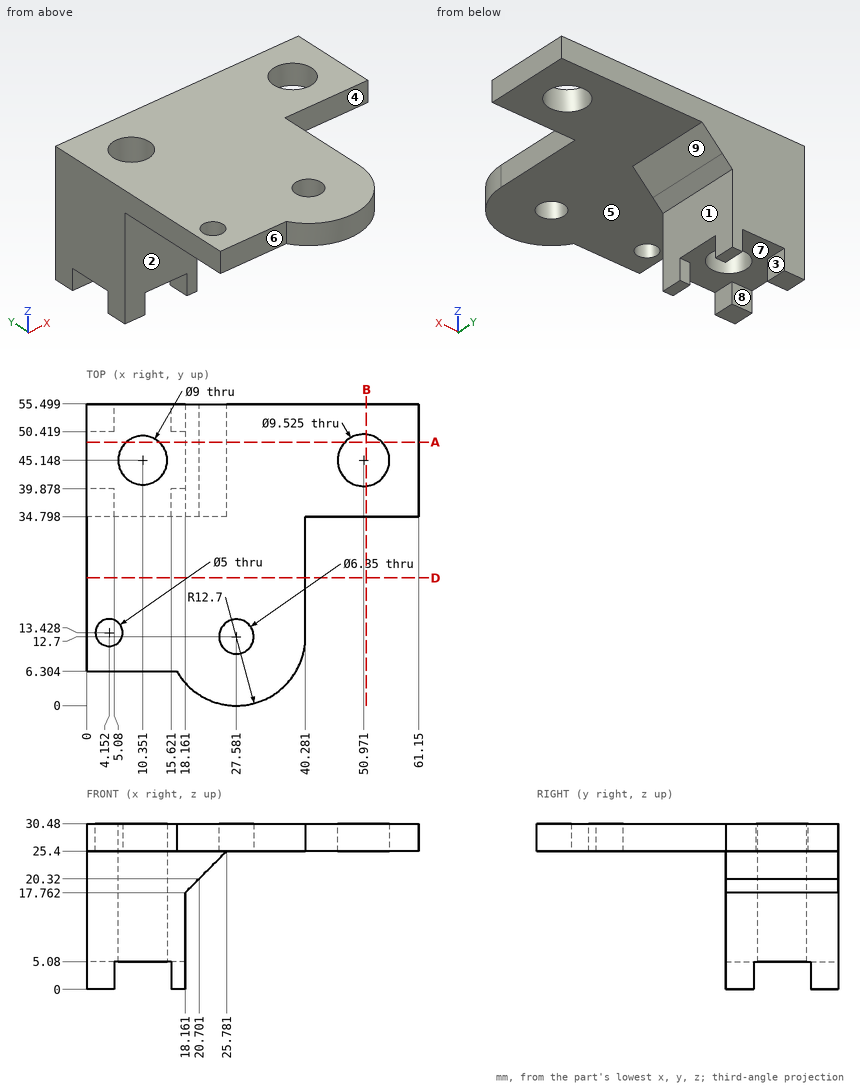
The drawing under review shows one solid part. Ordinate dimensions are in mm from its lowest x, y, z. A direction names the side the tool comes from. Round coordinates to 2 decimals unless told otherwise and drop trailing zeros. Write each loop counter-clockwise with the first axis right and the second up, starting at its lowest first coordinate (ties: lowest second). Pieces come first, ordered by that corner, then holes. Notation, with made-up numbers: M 31,64.25 L 35,64.25 A11 ccw 35,80.25 Z; hole C -8,-23.75 d6. An arc over 180 degrees is marked long. One line per item, written item: value. Start each with the question number.
(1) Insertion check: pin 1 (4 mm diameter, centred on y = 52.5, z = 1.5, fed in from +X); pin 2 (4 mm diameter, centred on x = 2, z = 3.5, fed in from -Y); pin 3 (14.5 mm diameter, centred on x = 10.35, y = 45.15, fed in from -Z); pin 4 (4 mm diameter, centred on x = 4.15, y = 13.43, fed in from +Z). Each pin has a flat end and moves straight along its axis. Give the tip position at first contact, or say it passes through.
(2) Machinability: for the marked faces 1, 2, 3, 4 and 5, which of the approach directions +Z, -Z, +X, -X, +Y, -Y give a long, thin tool a straight path to every point of the face, cutting with its end or side? Answer none if there is none.
(3) Wall thickness on line 1 (Y direction, x = 10, z = 23.5) (1 decimal); line 2 (Z direction, x = 30, y = 24); line 3 (Y direction, x = 30, z = 26) (1 decimal): over which ranges is each line inside the solid? List them lowest first.
(4) We need section D-D (y = 23.5). Give the boundary of the cut face in (x, z), and give its area (3 significant figures).
(5) We need section A-A (y = 48.5). Count the separate pieces of the cut face and the enclosed holes in it, and give its area (3 significant figures).
(6) We need section B-B (x = 51.5). Give the boundary of the cut face in (y, z) (1 decimal).
(7) The part is to be moulded in two halves that separate along Y. For the marked faces 6, 7, 8 and 9, say which applies: released by +Y, released by -Y, zero draft, split by the parting line, or undercut.
Result:
1. pin 1: x = 18.16
1. pin 2: y = 34.8
1. pin 3: z = 5.08
1. pin 4: through
2. face 1: -Z, +X, +Y, -Y
2. face 2: -Z, +X, -X, -Y
2. face 3: -Z, +Y, -Y
2. face 4: +Z, -Z, +X, -Y
2. face 5: -Z, +X, -Y
3. line 1: 34.8 to 40.7, 49.6 to 55.5
3. line 2: 25.4 to 30.48
3. line 3: 0.2 to 10.6, 14.8 to 55.5
4. outline: M 0,25.4 L 40.28,25.4 L 40.28,30.48 L 0,30.48 Z
4. area: 205 mm²
5. separate pieces: 3
5. enclosed holes: 0
5. area: 522 mm²
6. outline: M 34.8,25.4 L 40.4,25.4 L 40.4,30.5 L 34.8,30.5 Z; M 49.9,25.4 L 55.5,25.4 L 55.5,30.5 L 49.9,30.5 Z
7. face 6: released by -Y
7. face 7: undercut
7. face 8: undercut
7. face 9: zero draft
